from build123d import *

# Parameters (mm, degrees)
SKETCH1_W                                      = 76.2
SKETCH1_H                                      = 12.7
BOSS_EXTRUDE1_DEPTH                            = 3.175
F_5_16_CLEARANCE_HOLE1_D                       = 8.4328
F_5_16_CLEARANCE_HOLE1_DEPTH                   = 16.51
F_5_16_CLEARANCE_HOLE1_TIP                     = 2.533468714
BOSS_EXTRUDE2_DEPTH                            = 6.35
CBORE_FOR_8_SOCKET_HEAD_CAP_SCREW1_D           = 4.4958
CBORE_FOR_8_SOCKET_HEAD_CAP_SCREW1_DEPTH       = 16.51
CBORE_FOR_8_SOCKET_HEAD_CAP_SCREW1_CBORE_D     = 7.9375
CBORE_FOR_8_SOCKET_HEAD_CAP_SCREW1_CBORE_DEPTH = 4.1656
CBORE_FOR_8_SOCKET_HEAD_CAP_SCREW1_TIP         = 1.350674586
F_8_32_TAPPED_HOLE1_D                          = 3.4544
FILLET1_R                                      = 3.175


with BuildPart() as part:
    # Sketch1 → Boss-Extrude1 (new, symmetric)
    with BuildSketch(Plane(origin=(0, 0, 0), x_dir=(1, 0, 0), z_dir=(0, 1, 0))):
        Rectangle(SKETCH1_W, SKETCH1_H)
    extrude(amount=BOSS_EXTRUDE1_DEPTH, both=True)

    # 5/16 Clearance Hole1
    with Locations(Plane(origin=(0, 3.175, 0), x_dir=(1, 0, 0), z_dir=(0, 1, 0))):
        with Locations((0, 0)):
            Hole(F_5_16_CLEARANCE_HOLE1_D / 2, depth=F_5_16_CLEARANCE_HOLE1_DEPTH)
            with Locations((0, 0, -(F_5_16_CLEARANCE_HOLE1_DEPTH + F_5_16_CLEARANCE_HOLE1_TIP / 2))):  # 118° drill point
                Cone(0, F_5_16_CLEARANCE_HOLE1_D / 2, F_5_16_CLEARANCE_HOLE1_TIP, mode=Mode.SUBTRACT)

    # Sketch6 → Boss-Extrude2 (add, symmetric)
    with BuildSketch(Plane.XY):
        Polygon((38.1, 3.175), (32.907844009, 8.367155991), (27.715688019, 3.175), align=None)
    extrude(amount=BOSS_EXTRUDE2_DEPTH, both=True)

    # CBORE for #8 Socket Head Cap Screw1
    with Locations(Plane(origin=(0, -3.175, 0), x_dir=(-1, 0, 0), z_dir=(0, -1, 0))):
        with Locations((34.925, 0)):
            CounterBoreHole(CBORE_FOR_8_SOCKET_HEAD_CAP_SCREW1_D / 2, CBORE_FOR_8_SOCKET_HEAD_CAP_SCREW1_CBORE_D / 2, CBORE_FOR_8_SOCKET_HEAD_CAP_SCREW1_CBORE_DEPTH, depth=CBORE_FOR_8_SOCKET_HEAD_CAP_SCREW1_DEPTH)
            with Locations((0, 0, -(CBORE_FOR_8_SOCKET_HEAD_CAP_SCREW1_DEPTH + CBORE_FOR_8_SOCKET_HEAD_CAP_SCREW1_TIP / 2))):  # 118° drill point
                Cone(0, CBORE_FOR_8_SOCKET_HEAD_CAP_SCREW1_D / 2, CBORE_FOR_8_SOCKET_HEAD_CAP_SCREW1_TIP, mode=Mode.SUBTRACT)

    # #8-32 Tapped Hole1 (through all)
    with Locations(Plane(origin=(12.270344009, -12.270344009, 0), x_dir=(0.7071067811865476, 0.7071067811865475, 0), z_dir=(-0.7071067811865475, 0.7071067811865476, 0))):
        with Locations((26.010832393, 0)):
            Hole(F_8_32_TAPPED_HOLE1_D / 2)

    # Fillet1
    fillet1_edges = [part.edges().sort_by_distance(p)[0] for p in [
        (27.715688019, 3.175, 0),
    ]]
    fillet(fillet1_edges, radius=FILLET1_R)


solid = part.part
Here's how the part is built. I have some questions about the finished solid (model axes, mm). A direction names the side the tool comes from. Round coordinates to 2 decimals unless told otherwise and drop trailing zeros. Write each loop counter-clockwise with the first axis right and the second up, starting at its lowest first coordinate (ties: lowest second). Pieces come first, ordered by that corner, then holes.
1. Suppose I cut it at C-C (x = 17). List the corners of the cut face in (y, z) for me (3 decimals), and give its area (3 significant figures).
2. I need wall thicknesses on L1, parallel to Z at x = 0, y = 1.25; L2, parallel to X at y = 0.5, z = -3.25; L3, parallel to Y at x = -11, z = -4.5 (3 decimals). Which ranges of each line are inside material? Lowest first, please.
3. Will these pins go through, and if not, where does the flat tip stop? pin 1 Ø3 at (y, z) = (7, -5) entering from +X (3 decimals); pin 2 Ø5 at (x, z) = (-34.925, 0) entering from -Y; pin 3 Ø6 at (x, z) = (-34.925, 0) entering from +Y (3 decimals); pin 4 Ø6.5 at (x, z) = (0, 0) entering from -Y.
4. For faces 1 (the flat face through (38.1, 1.5, 0.1)), 2 (the cylindrical face through (-30.96, -1.12, -0.14)), 3 (the flat face through (-6, 3.175, 0)), which set-ups out of +Z, -Z, +X, -X, +Y, -Y let a thin tool reach every point of the face, with its end or its side?
5. Suppose I cut it at B-B (z = 0). State how many separate pieces and enclosed holes the cut face has, and give its area (3 significant figures).
6. If we mould it in two halves opening along X, with no side actions, what happens to faces 4 (the flat face through (-33, 0.991, 2)), 5 (the flat face through (8, -3.175, 0)), 6 (the flat face through (31.75, 7.21, 1.5))? For each: released by +X, released by -X, zero draft, split by the parting line, or undercut.
7. Suppose I cut it at A-A (x = 0). List the corners of the cut face in (y, z) for me (3 decimals).
Answer sheet:
1. outline: (-3.175, -6.35) - (3.175, -6.35) - (3.175, 6.35) - (-3.175, 6.35) - close
1. area: 80.6 mm2
2. L1: z = -6.35 to -4.22, 4.22 to 6.35
2. L2: x = -38.1 to -37.2, -32.65 to -2.69, 2.69 to 38.1
2. L3: y = -3.175 to 3.175
3. pin 1: stops at x = 35.775
3. pin 2: stops at y = 0.99
3. pin 3: stops at y = 3.175
3. pin 4: passes through
4. face 1: +Z, -Z, +X, +Y, -Y
4. face 2: -Y
4. face 3: +Z, -Z, -X, +Y
5. separate pieces: 4
5. enclosed holes: 0
5. area: 382 mm2
6. face 4: undercut
6. face 5: zero draft
6. face 6: released by -X
7. outline: (-3.175, -6.35) - (3.175, -6.35) - (3.175, -4.216) - (-3.175, -4.216) - close; (-3.175, 4.216) - (3.175, 4.216) - (3.175, 6.35) - (-3.175, 6.35) - close
